Read the model definition and answer for the solid it produces. Units are mm, in the model's axes. A direction names the side the tool comes from. Coordinates: 2 decimals unless noted, no trailing zeros. Order: outer loops, then holes, each group sorted by start corner. A loop starts at its lowest first (then second) coordinate and runs counter-clockwise, first axis right, second up. Notation, with made-up numbers: (-32.5, 47) -> (-18.5, 47) arc R3 cw to (-18.5, 52) -> close; hole circle Ø8 at (45, 1.25). An arc over 180 degrees is marked (long way). Answer as a JSON object with one key per item and string values. Group by question number.
1) Given pin 1 (1.5 mm diameter, centred on x = -8, z = 47.5, fed in from -Y); pin 2 (6.5 mm diameter, centred on x = 0, y = 0, fed in from +Z); pin 3 (5 mm diameter, centred on y = -4.5, z = 37.5, fed in from +X); pin 4 (1 mm diameter, centred on x = -2, z = 44, fed in from +Y), each flat-ended and moving along its own axis, determine where each tip first touches the part or whether it passes through.
2) Determine the mould class of faces 3 (the cylindrical face through (-3.19, -14.35, 1.01)), 4 (the flat face through (3, -3, 0)), 5 (the flat face through (-13, 0, 67.85)), 6 (the flat face through (3, -3, 69.85)) for opening direction Z: released by +Z, released by -Z, zero draft, split by the parting line, or undercut.
3) Section A-A on y = 0 is taken. Determine the outline of the cut face in (x, z).
4) Section C-C on x = -8.75 is taken. Determine the outline of the cut face in (y, z), and give its area (3 significant figures).
5) Section D-D on z = 29 is taken. Determine the outline of the cut face in (x, y).
6) Consider L1, parallel to Z at x = -9.25, y = 11.25; L2, parallel to Y at x = 0, z = 48; L3, parallel to Y at x = -1.25, z = 52.5. Determine where each line is inside the solid, lowest interval first.
7) A tool of negligible diameter and unlimited length cuts with its end or side. For faces 1 (the cylindrical face through (-3.19, -14.35, 68.86)), 2 (the cylindrical face through (-2.75, -12.4, 34.46)), from which of +Z, -Z, +X, -X, +Y, -Y can it reach the whole face along a straight path? Write none if from no direction.
from build123d import *

# Parameters (mm, degrees)
SKETCH1_R           = 12.7
BOSS_EXTRUDE1_DEPTH = 69.85
SKETCH2_R           = 3.572
CUT_EXTRUDE3_DEPTH  = 69.85
BOSS_EXTRUDE2_START = 2
SKETCH3_R           = 14.7
SKETCH3_R_2         = 3.572
BOSS_EXTRUDE2_DEPTH = 2
BOSS_EXTRUDE3_START = 69.85
SKETCH3_2_R         = 14.7
SKETCH3_2_R_2       = 3.572
BOSS_EXTRUDE3_DEPTH = 2


with BuildPart() as part:
    # Sketch1 → Boss-Extrude1 (new body)
    with BuildSketch(Plane.XY):
        Circle(SKETCH1_R)
    extrude(amount=BOSS_EXTRUDE1_DEPTH)

    # Sketch2 → Cut-Extrude3 (cut)
    with BuildSketch(Plane.XY.offset(69.85)):
        Circle(SKETCH2_R)
    extrude(amount=-CUT_EXTRUDE3_DEPTH, mode=Mode.SUBTRACT)

    # Sketch3 → Boss-Extrude2 (add)
    with BuildSketch(Plane.XY.offset(BOSS_EXTRUDE2_START)):
        Circle(SKETCH3_R)
        Circle(SKETCH3_R_2, mode=Mode.SUBTRACT)
    extrude(amount=-BOSS_EXTRUDE2_DEPTH)

    # Sketch3<2> → Boss-Extrude3 (add)
    with BuildSketch(Plane.XY.offset(BOSS_EXTRUDE3_START)):
        Circle(SKETCH3_2_R)
        Circle(SKETCH3_2_R_2, mode=Mode.SUBTRACT)
    extrude(amount=-BOSS_EXTRUDE3_DEPTH)


solid = part.part
Worked answers:
{
 "1": {"pin 1": "stops at y = -10.43", "pin 2": "passes through", "pin 3": "stops at x = 12.54", "pin 4": "stops at y = 12.61"},
 "2": {"face 3": "zero draft", "face 4": "released by -Z", "face 5": "undercut", "face 6": "released by +Z"},
 "3": {"outline": "(-14.7, 0) -> (-3.57, 0) -> (-3.57, 69.85) -> (-14.7, 69.85) -> (-14.7, 67.85) -> (-12.7, 67.85) -> (-12.7, 2) -> (-14.7, 2) -> close; (3.57, 0) -> (14.7, 0) -> (14.7, 2) -> (12.7, 2) -> (12.7, 67.85) -> (14.7, 67.85) -> (14.7, 69.85) -> (3.57, 69.85) -> close"},
 "4": {"outline": "(-11.81, 0) -> (11.81, 0) -> (11.81, 2) -> (9.2, 2) -> (9.2, 67.85) -> (11.81, 67.85) -> (11.81, 69.85) -> (-11.81, 69.85) -> (-11.81, 67.85) -> (-9.2, 67.85) -> (-9.2, 2) -> (-11.81, 2) -> close", "area": "1,310 mm²"},
 "5": {"outline": "circle Ø25.4 at (0, 0); hole circle Ø7.14 at (0, 0)"},
 "6": {"L1": "z = 0 to 2, 67.85 to 69.85", "L2": "y = -12.7 to -3.57, 3.57 to 12.7", "L3": "y = -12.64 to -3.35, 3.35 to 12.64"},
 "7": {"face 1": "+Z, -Z", "face 2": "none"}
}
